Input: part model. Units: mm. Frame: model coordinates. Face numbers are marked on the shaded views. A direction names the side the tool comes from. Round coordinates to 2 decimals unless told otherwise and drop trailing zeros. Loops run counter-clockwise (first coordinate to the right, second up) from the corner with the lowest first, then second, coordinate; pieces in that order, holes last.
1) Section B-B, the plane x = 0. Return loops of the section in (y, z).
2) Section D-D, the plane x = -5.5. Return loops of the section in (y, z).
3) Ray query, line 1 along X through (y, z) = (0.15, 0); line 2 along X through (y, z) = (-10.5, 1.25); line 3 along Y through (x, z) = (2.75, 0.5). Return the intervals inside material, ascending.
4) Section A-A, the plane y = -8. Return loops of the section in (x, z), and give its area (3 significant figures).
5) Draft query along Z for the marked faces 1, 2, 3 and 4. Return one class per face: pulls with the +Z half, pulls with the -Z half, needs draft (parallel to the pull), parting line crosses it, or undercut.
6) First-contact query: pin 1 (1.5 mm diameter, centred on x = -5, z = 0.5, fed in from +Y); pin 2 (3 mm diameter, centred on y = -16, z = -4.5, fed in from +X); pin 3 (1.4 mm diameter, centred on x = -7, y = -7.5, fed in from -Z). Flat tips, straight axial feed; report the tip coordinate or a pass-through.
7) Access query for the marked faces 5 and 6. Directions: +Z, -Z, +X, -X, +Y, -Y. A direction counts if a zero-diameter tool reaches every point of the face in a straight line with its end or side. Return the directions, or none.
8) Section C-C, the plane z = 0. State how many separate pieces and enclosed holes the cut face has, and give its area (3 significant figures).
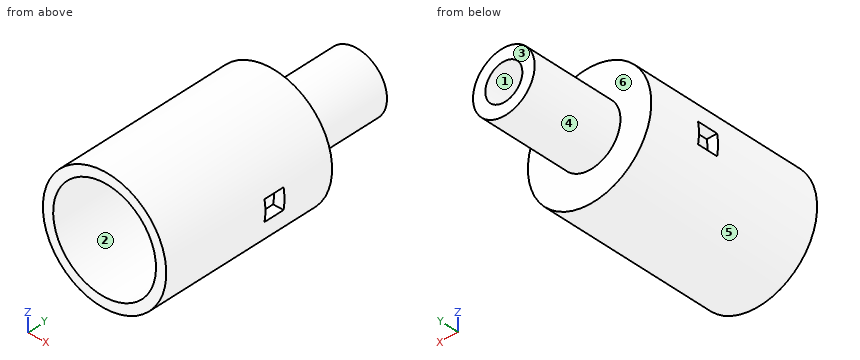
from build123d import *

# Parameters (mm, degrees)
SKETCH2_R                = 7.62
BOSS_EXTRUDE1_DEPTH      = 22.098
SKETCH3_R                = 6.35
CUT_EXTRUDE1_DEPTH       = 16.764
CUT_EXTRUDE3_DEPTH       = 16.764
CUT_EXTRUDE3_DEPTH_BACK  = 25.585573087
SKETCH5_R                = 2.3495
SKETCH6_R                = 3.81
BOSS_EXTRUDE2_DEPTH      = 11.43
SKETCH8_R                = 2.286
CUT_EXTRUDE4_DEPTH       = 11.176
CUT_EXTRUDE8_REACH       = 26.586
SKETCH10_R               = 1.719833609
CUT_EXTRUDE10_DEPTH      = 25.585573087
CUT_EXTRUDE10_DEPTH_BACK = 25.585573087
SKETCH12_W               = 2.54
SKETCH12_H               = 2.54


with BuildPart() as part:
    # Sketch2 → Boss-Extrude1 (new body)
    with BuildSketch(Plane(origin=(0, 0, 0), x_dir=(1, 0, 0), z_dir=(0, 1, 0))):
        with Locations(Location((0, 0, 0), (0, 0, 270))):
            Circle(SKETCH2_R)
    extrude(amount=-BOSS_EXTRUDE1_DEPTH)

    # Sketch3 → Cut-Extrude1 (cut)
    with BuildSketch(Plane.XZ.offset(22.098)):
        with Locations(Location((0, 0, 0), (0, 0, 270))):
            Circle(SKETCH3_R)
    extrude(amount=-CUT_EXTRUDE1_DEPTH, mode=Mode.SUBTRACT)

    # Sketch5 → Cut-Extrude3 (cut, two sides: drawn at the far end of the back side and taken through both)
    with BuildSketch(Plane(origin=(0, 0, 0), x_dir=(1, 0, 0), z_dir=(0, 1, 0)).offset(-CUT_EXTRUDE3_DEPTH_BACK)):
        with Locations(Location((0, 0, 0), (0, 0, 270))):
            Circle(SKETCH5_R)
    extrude(amount=CUT_EXTRUDE3_DEPTH + CUT_EXTRUDE3_DEPTH_BACK, mode=Mode.SUBTRACT)

    # Sketch6 → Boss-Extrude2 (add)
    with BuildSketch(Plane(origin=(0, 0, 0), x_dir=(1, 0, 0), z_dir=(0, 1, 0))):
        with Locations(Location((0, 0, 0), (0, 0, 270))):
            Circle(SKETCH6_R)
    extrude(amount=BOSS_EXTRUDE2_DEPTH)

    # Sketch8 → Cut-Extrude4 (cut)
    with BuildSketch(Plane(origin=(0, 11.43, 0), x_dir=(1, 0, 0), z_dir=(0, 1, 0))):
        with Locations(Location((0, 0, 0), (0, 0, 270))):
            Circle(SKETCH8_R)
    extrude(amount=-CUT_EXTRUDE4_DEPTH, mode=Mode.SUBTRACT)

    # Sketch10 → Cut-Extrude8 (cut, up to next)
    with BuildSketch(Plane.XZ, mode=Mode.PRIVATE) as cut_extrude8_sk1:
        with Locations(Location((0, 0, 0), (0, 0, 270))):
            Circle(SKETCH10_R)
    cut_extrude8_tool1 = extrude(cut_extrude8_sk1.sketch, amount=-CUT_EXTRUDE8_REACH, mode=Mode.PRIVATE) & part.part
    add(cut_extrude8_tool1.solids().sort_by_distance((0, 0, 0))[0], mode=Mode.SUBTRACT)

    # Sketch12 → Cut-Extrude10 (cut, two sides: drawn at the far end of the back side and taken through both)
    with BuildSketch(Plane(origin=(0, 0, 0), x_dir=(0, 0, -1), z_dir=(1, 0, 0)).offset(-CUT_EXTRUDE10_DEPTH_BACK)):
        with Locations((0, -7.62)):
            Rectangle(SKETCH12_W, SKETCH12_H)
    extrude(amount=CUT_EXTRUDE10_DEPTH + CUT_EXTRUDE10_DEPTH_BACK, mode=Mode.SUBTRACT)


solid = part.part
Final values:
1. outline: (-22.1, -7.62) - (0, -7.62) - (0, -3.81) - (11.43, -3.81) - (11.43, -2.29) - (0.25, -2.29) - (0.25, -1.72) - (0, -1.72) - (0, -2.35) - (-5.33, -2.35) - (-5.33, -6.35) - (-22.1, -6.35) - close; (-22.1, 6.35) - (-5.33, 6.35) - (-5.33, 2.35) - (0, 2.35) - (0, 1.72) - (0.25, 1.72) - (0.25, 2.29) - (11.43, 2.29) - (11.43, 3.81) - (0, 3.81) - (0, 7.62) - (-22.1, 7.62) - close
2. outline: (-22.1, -5.27) - (0, -5.27) - (0, 5.27) - (-22.1, 5.27) - (-22.1, 3.17) - (-5.33, 3.17) - (-5.33, -3.17) - (-22.1, -3.17) - close
3. line 1: x = -3.81 to -1.72, 1.72 to 3.81
3. line 2: x = -7.52 to -6.23, 6.23 to 7.52
3. line 3: y = -5.33 to 11.43
4. outline: (-7.51, -1.27) arc R7.62 ccw to (7.51, -1.27) - (6.22, -1.27) arc R6.35 cw to (-6.22, -1.27) - close; (-7.51, 1.27) - (-6.22, 1.27) arc R6.35 cw to (6.22, 1.27) - (7.51, 1.27) arc R7.62 ccw to start
4. area: 49.2 mm2
5. face 1: undercut
5. face 2: undercut
5. face 3: needs draft
5. face 4: parting line crosses it
6. pin 1: stops at y = 0
6. pin 2: stops at x = 7
6. pin 3: stops at z = -4.29
7. face 5: +Y, -Y
7. face 6: +Y
8. separate pieces: 4
8. enclosed holes: 0
8. area: 127 mm2
